from build123d import *

# Parameters (mm, degrees)
RESSALTO_EXTRUS_O1_DEPTH = 70
CORTE_EXTRUS_O1_DEPTH    = 70


with BuildPart() as part:
    # Esboço1 → Ressalto-extrusão1 (new body)
    with BuildSketch(Plane.XY):
        Polygon((-46.166666667, -15.652777778), (33.833333333, 19.347222222), (33.833333333, -15.652777778), align=None)
    extrude(amount=RESSALTO_EXTRUS_O1_DEPTH)

    # Esboço2 → Corte-extrusão1 (cut)
    with BuildSketch(Plane.XZ.offset(15.652777778)):
        with BuildLine():
            Line((-11.166666667, 0), (-1.166666667, 0))
            Line((-1.166666667, 0), (-1.166666667, 5.846688069))
            ThreePointArc((-1.166666667, 5.846688069), (-6.166666667, 16.5), (-11.166666667, 5.846688069))
            Line((-11.166666667, 5.846688069), (-11.166666667, 0))
        make_face()
    extrude(amount=-CORTE_EXTRUS_O1_DEPTH, mode=Mode.SUBTRACT)


solid = part.part
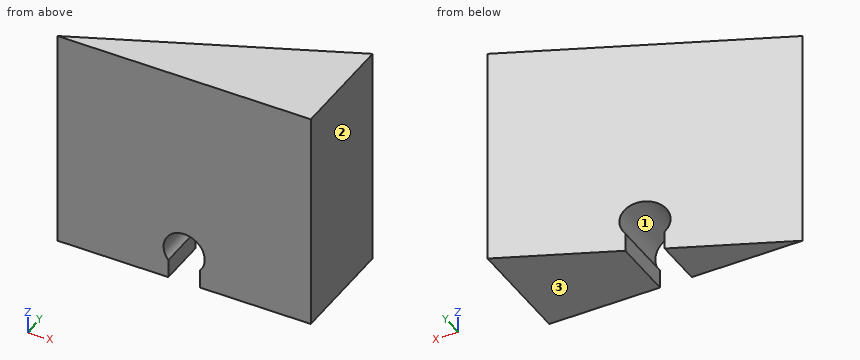
Source: CAD feature listing. Evaluate the final solid. Frame: model axes, mm. Face numbers are marked on the shaded views. Coordinates: 2 decimals unless noted, no trailing zeros. Loops run counter-clockwise (first coordinate to the right, second up) from the corner with the lowest first, then second, coordinate; pieces in that order, holes last. Notation, with made-up numbers: (88, -29.75) - (142, -29.75) arc R13 ccw to (142, -13.75) - close; hole circle Ø7 at (60, 49). An arc over 180 degrees is marked (long way). One line per item, written item: value. Start each with the question number.
1. Section A-A (z = 10). Return the cut outline in (x, y).
2. Section D-D (x = -4.5). Return the cut outline in (y, z).
3. Section B-B (y = 2). Return the cut outline in (x, z).
4. Ray query, L1, parallel to X at y = -10.75, z = 10; L2, parallel to X at y = -3.25, z = 10; L3, parallel to Y at x = 5.5, z = 58.5. Return the intervals inside material, ascending.
5. Contact query for flat-ended pins moving along their axis: P1, Ø12, axis at x = 3, z = 17.5, coming from the +Y side; P2, Ø5, axis at y = 3, z = 36.5, coming from the -X side; P3, Ø3, axis at y = -9, z = 2.5, coming from the -X side. Output: stop coordinate, or through.
6. Mould query, pull axis Z, two halves, no side actions, for the marked faces 1, 2 and 3. Classes: pulls with the +Z half, pulls with the -Z half, needs draft (parallel to the pull), parting line crosses it, or undercut.
7. Section C-C (z = 58). Return the cut outline in (x, y), and give its area (3 significant figures).
Verdict:
1. outline: (-46.17, -15.65) - (-12.67, -15.65) - (-12.67, -1) - close; (0.33, -15.65) - (33.83, -15.65) - (33.83, 19.35) - (0.33, 4.69) - close
2. outline: (-15.65, 16.28) - (2.58, 16.28) - (2.58, 70) - (-15.65, 70) - close
3. outline: (-5.82, 16.49) arc R6.5 cw to (-1.17, 5.85) - (-1.17, 0) - (33.83, 0) - (33.83, 70) - (-5.82, 70) - close
4. L1: x = -34.96 to -12.67, 0.33 to 33.83
4. L2: x = -17.82 to -12.67, 0.33 to 33.83
4. L3: y = -15.65 to 6.95
5. P1: stops at y = 8.48
5. P2: stops at x = -9.25
5. P3: stops at x = -34.39
6. face 1: undercut
6. face 2: needs draft
6. face 3: pulls with the -Z half
7. outline: (-46.17, -15.65) - (33.83, -15.65) - (33.83, 19.35) - close
7. area: 1,400 mm2
